Read the model definition and answer for the solid it produces. Units are mm, in the model's axes. A direction names the side the tool comes from. Round coordinates to 2 decimals unless told otherwise and drop trailing zeros. Order: outer loops, then holes, each group sorted by start corner. A loop starts at its lowest first (then second) coordinate and runs counter-clockwise, first axis right, second up. Notation, with made-up numbers: (85, 25.5) -> (124, 25.5) arc R18 ccw to (124, 39.5) -> close; hole circle Ø6 at (3.25, 42.25). An arc over 180 degrees is marked (long way). Answer as a JSON object with one key per item and string values. Group by question number.
Item 1: For faces 1 (the flat face through (0, 2.5, 81)), 2 (the flat face through (0, 3, 165)), determine the directions among +Z, -Z, +X, -X, +Y, -Y from which every point of the face is accessible in a straight line to the end or side of a thin tool.
Item 2: Section A-A, the plane x = -0.75 is taken. Write down the section's boundary in (y, z), plus the area to 4 significant figures.
Item 3: Section C-C, the plane z = 39 is taken. Write down the section's boundary in (x, y).
Item 4: Given P1, Ø3, axis at x = -1, y = -2, coming from the -Z side, flat-ended and moving along its own axis, determine where the tip first touches the part or whether it passes through.
Item 5: Consider probe 1 along Y at (x, z) = (1.75, 74.5); probe 2 along X at (y, z) = (3.5, 52.5). Determine where each line is inside the solid, lowest interval first. Write a range as from..to.
Item 6: The mould has two halves that part along X. Classify faces 3 (the flat face through (-3.75, 0, 81)), 4 (the flat face through (2.5, 0, 81)), 5 (the flat face through (0, 3.75, 81)): pulls with the +X half, pulls with the -X half, needs draft (parallel to the pull), parting line crosses it, or undercut.
Autodesk Inventor part; units mm, degrees
ref_plane "YZ Plane" through (0, 0, 0) normal (1, 0, 0) x (0, 1, 0)
ref_plane "XZ Plane" through (0, 0, 0) normal (0, 1, 0) x (-1, 0, 0)
ref_plane "XY Plane" through (0, 0, 0) normal (0, 0, 1) x (1, 0, 0)
sketch "Sketch1" plane through (0, 0, 0) normal (0, 0, 1) x (1, 0, 0)
  circle A0 centre (0, 0) radius 5
  line L0 (-2.5, 2.5) -> (2.5, 2.5)
  line L1 (2.5, 2.5) -> (2.5, -2.5)
  line L2 (2.5, -2.5) -> (-2.5, -2.5)
  line L3 (-2.5, -2.5) -> (-2.5, 2.5)
  line L4 (-2.5, 2.5) -> (2.5, -2.5) construction
  line L5 (2.5, 2.5) -> (-2.5, -2.5) construction
  line L6 (-3.75, 3.75) -> (3.75, 3.75)
  line L7 (3.75, 3.75) -> (3.75, -3.75)
  line L8 (3.75, -3.75) -> (-3.75, -3.75)
  line L9 (-3.75, -3.75) -> (-3.75, 3.75)
  line L10 (-3.75, 3.75) -> (3.75, -3.75) construction
  line L11 (3.75, 3.75) -> (-3.75, -3.75) construction
  point P0 (-3.75, 3.3072)
  point P1 (-3.75, -3.3072)
  point P2 (-3.3072, -3.75)
  point P3 (3.3072, -3.75)
  point P4 (3.75, -3.3072)
  point P5 (3.75, 3.3072)
  point P6 (3.3072, 3.75)
  point P7 (-3.3072, 3.75)
  dimension "d0" = 10
  dimension "d1" = 5
  dimension "d2" = 5
  dimension "d3" = 7.5
  dimension "d4" = 7.5
extrude "Extrusion1" add sketch "Sketch1" along normal blind 165 contours L7 A0 L8 L9 L6
properties part number "IgusDryLinQ-AWMQ-10" material "Aluminum 6061"
Values found:
{
 "1": {"face 1": "+Z, -Z", "face 2": "+Z, +X, -X, +Y, -Y"},
 "2": {"outline": "(-3.75, 0) -> (-2.5, 0) -> (-2.5, 165) -> (-3.75, 165) -> close; (2.5, 0) -> (3.75, 0) -> (3.75, 165) -> (2.5, 165) -> close", "area": "412.5 mm2"},
 "3": {"outline": "(-3.75, -3.31) arc R5 ccw to (-3.31, -3.75) -> (3.31, -3.75) arc R5 ccw to (3.75, -3.31) -> (3.75, 3.31) arc R5 ccw to (3.31, 3.75) -> (-3.31, 3.75) arc R5 ccw to (-3.75, 3.31) -> close; hole (-2.5, -2.5) -> (2.5, -2.5) -> (2.5, 2.5) -> (-2.5, 2.5) -> close"},
 "4": {"P1": "z = 0"},
 "5": {"probe 1": "-3.75..-2.5, 2.5..3.75", "probe 2": "-3.57..3.57"},
 "6": {"face 3": "pulls with the -X half", "face 4": "undercut", "face 5": "needs draft"}
}
